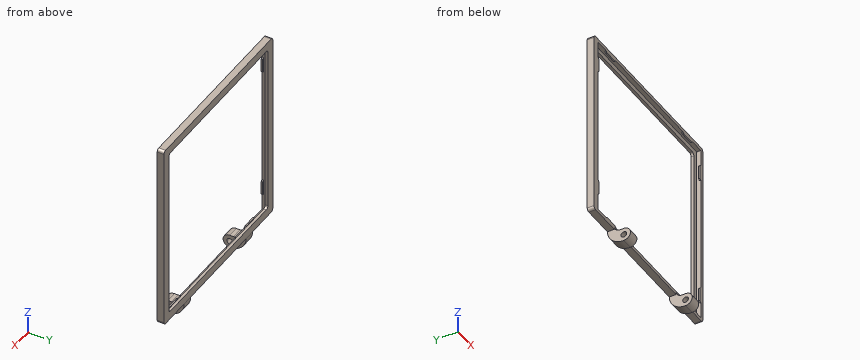
Autodesk Inventor part; units mm, degrees
ref_plane "YZ Plane" through (0, 0, 0) normal (1, 0, 0) x (0, 1, 0)
ref_plane "XZ Plane" through (0, 0, 0) normal (0, 1, 0) x (-1, 0, 0)
ref_plane "XY Plane" through (0, 0, 0) normal (0, 0, 1) x (1, 0, 0)
sketch "Boceto1" plane through (0, 0, 0) normal (0, 1, 0) x (-1, 0, 0)
  line L0 (2, 0) -> (132.4, 0)
  line L1 (134.4, -2) -> (134.4, -138)
  line L2 (132.4, -140) -> (2, -140)
  line L3 (0, -138) -> (0, -2)
  arc A0 (134.4, -2) -> (132.4, 0) centre (132.4, -2) ccw
  arc A1 (132.4, -140) -> (134.4, -138) centre (132.4, -138) ccw
  arc A2 (0, -138) -> (2, -140) centre (2, -138) ccw
  arc A3 (2, 0) -> (0, -2) centre (2, -2) ccw
  line L4 (126.4, -6) -> (8, -6)
  line L5 (6, -8) -> (6, -132)
  line L6 (8, -134) -> (126.4, -134)
  line L7 (128.4, -132) -> (128.4, -8)
  arc A4 (8, -6) -> (6, -8) centre (8, -8) ccw
  arc A5 (6, -132) -> (8, -134) centre (8, -132) ccw
  arc A6 (126.4, -134) -> (128.4, -132) centre (126.4, -132) ccw
  arc A7 (128.4, -8) -> (126.4, -6) centre (126.4, -8) ccw
  line L8 (67.2, -140) -> (67.2, 0) construction
  line L9 (134.4, -140) -> (109.4, -140) construction
  line L10 (109.4, -140) -> (101.4, -140) construction
  line L11 (101.4, -140) -> (101.4, -152)
  line L12 (101.4, -152) -> (109.4, -152)
  line L13 (109.4, -152) -> (109.4, -140)
  line L14 (0, -140) -> (25, -140) construction
  line L15 (25, -140) -> (33, -140) construction
  line L16 (33, -140) -> (33, -152)
  line L17 (33, -152) -> (25, -152)
  line L18 (25, -152) -> (25, -140)
  point P0 (0, 0)
  point P1 (134.4, 0)
  point P2 (25, -140)
  point P3 (101.4, -140)
  dimension "d0" = 134.4
  dimension "d1" = 140
  dimension "d2" = 2
  dimension "d3" = 6
  dimension "d4" = 2
  dimension "d7" = 25
  dimension "d8" = 8
  dimension "d9" = 12
extrude "Extrusión1" add sketch "Boceto1" along normal blind 5
sketch "Boceto2" plane through (0, 0, 0) normal (0, -1, 0) x (1, 0, 0)
  line L0 (-25, -140) -> (-25, -152)
  line L1 (-33, -140) -> (-101.4, -140)
  line L2 (-25, -152) -> (-33, -152)
  line L3 (-33, -152) -> (-33, -140)
  line L4 (-33, -140) -> (-25, -140)
  line L5 (-25, -140) -> (-25, -152)
  line L6 (-101.4, -152) -> (-109.4, -152)
  line L7 (-109.4, -152) -> (-101.4, -152)
  line L8 (-101.4, -152) -> (-101.4, -140)
  line L9 (-101.4, -140) -> (-109.4, -140)
  line L10 (-109.4, -140) -> (-109.4, -152)
  line L11 (-109.4, -140) -> (-101.4, -140)
  line L12 (-101.4, -140) -> (-101.4, -136)
  line L13 (-101.4, -136) -> (-109.4, -136)
  line L14 (-109.4, -136) -> (-109.4, -140)
  line L15 (-33, -140) -> (-25, -140)
  line L16 (-25, -140) -> (-25, -136)
  line L17 (-25, -136) -> (-33, -136)
  line L18 (-33, -136) -> (-33, -140)
  point P0 (0, 0)
  dimension "d18" = 4
  dimension "d19" = 8
  dimension "d20" = 4
extrude "Extrusión2" add sketch "Boceto2" along normal blind 18
sketch "Boceto3" plane through (-109.4, 5, -152) normal (-1, 0, 0) x (0, 0, 1)
  line L0 (14, -5) -> (12, -5) construction
  line L1 (0, -23) -> (0, 0)
  line L2 (12, -5) -> (0, -5) construction
  line L3 (0, -5) -> (0, -12) construction
  line L4 (12, -12) -> (12, -5) construction
  circle A0 centre (5, -12) radius 2.125
  circle A1 centre (5, -12) radius 4.875 construction
  arc A2 (0.125, -12) -> (9.875, -12) centre (5, -12) ccw
  line L5 (0.125, -12) -> (0.125, 0) construction
  line L6 (12, 0) -> (0, 0) construction
  line L7 (12, -5) -> (12, 0) construction
  line L8 (9.8743, -12.0803) -> (9.8743, -5) construction
  line L9 (12, -5) -> (5, -5) construction
  line L10 (5, -5) -> (5, -12) construction
  line L11 (5, -12) -> (12, -12) construction
  line L12 (12, -12) -> (12, -5) construction
  line L13 (14, -5) -> (14, -23) construction
  line L14 (16, -23) -> (0, -23)
  line L15 (12, -5) -> (14, -5) construction
  line L16 (14, -5) -> (14, -7) construction
  line L17 (14, -7) -> (12, -7) construction
  line L18 (12, -7) -> (12, -5) construction
  arc A3 (14, -5) -> (12, -7) centre (14, -7) ccw construction
  line L19 (14, 0) -> (150, 0)
  line L20 (12, 0) -> (14, 0)
  arc A4 (12, 0) -> (0.125, -12) centre (12, -11.8757) ccw
  line L21 (14, -5) -> (16, -5)
  arc A5 (14, -5) -> (9.8743, -9.1856) centre (14, -9.1261) ccw
  line L22 (9.8743, -12.0803) -> (9.8743, -9.1856)
  line L23 (0.125, 0) -> (14, 0)
  line L24 (14, 0) -> (14, -23)
  line L25 (14, -23) -> (0, -23)
  line L26 (16, -23) -> (14, -23)
  line L27 (14, -23) -> (14, -5)
  line L28 (14, -5) -> (16, -5)
  line L29 (16, -5) -> (16, -23)
  line L30 (0.125, 0) -> (-6.5711, 0)
  line L31 (-6.5711, 0) -> (-6.5711, -23)
  line L32 (-6.5711, -23) -> (16, -23)
  point P0 (152, -5)
  point P1 (9.8743, -9.1856)
  point P2 (9.8743, -12.0803)
  point P3 (0, -10.3846)
  point P4 (0, -13.125)
  point P5 (12, 0)
  point P6 (0, 0)
  point P7 (14, -5)
  point P8 (14, -5)
  dimension "d13" = 4.25
  dimension "d14" = 2.75
  dimension "d16" = 7
  dimension "d17" = 7
  dimension "d21" = 2
extrude "Extrusión3" cut sketch "Boceto3" against normal blind 150 contours L1 L30 L23 A4 A2 L22 A5 L24 L14 | L24 L21 L29 L14 | A0
sketch "Boceto4" plane through (0, 0, 0) normal (0, -1, 0) x (1, 0, 0)
  line L0 (0, 0) -> (-132, 0)
  line L1 (-132, 0) -> (-132, -140)
  line L2 (-132, -140) -> (0, -140)
  line L3 (0, -140) -> (0, 0)
  line L4 (-2.5, -2.5) -> (-129.5, -2.5)
  line L5 (-129.5, -2.5) -> (-129.5, -137.5)
  line L6 (-129.5, -137.5) -> (-2.5, -137.5)
  line L7 (-2.5, -137.5) -> (-2.5, -2.5)
  dimension "d27" = 132
  dimension "d28" = 140
  dimension "d29" = 2.5
extrude "Extrusión4" cut sketch "Boceto4" against normal blind 3 contours L7 L6 L5 L4
sketch "Boceto5" plane through (0, 0, 0) normal (0, -1, 0) x (1, 0, 0)
  line L0 (-129.5, -137.5) -> (-129.5, -2.5)
  line L1 (-2.5, -2.5) -> (-2.5, -137.5)
  line L2 (-129.5, -137.5) -> (-2.5, -137.5)
  line L3 (-2.5, -137.5) -> (-2.5, -2.5)
  line L4 (-2.5, -2.5) -> (-129.5, -2.5)
  line L5 (-129.5, -2.5) -> (-129.5, -137.5)
  line L6 (-2.5, -137.5) -> (-129.5, -137.5)
  line L7 (-66, -137.5) -> (-66, -2.5) construction
  line L8 (-33, -140) -> (-101.4, -140) construction
  line L9 (-2.5, -70) -> (-129.5, -70) construction
  line L10 (-118.5, -137.5) -> (-107.5, -137.5) construction
  line L11 (-118.5, -137.5) -> (-108.5, -137.5) construction
  line L12 (-108.5, -137.5) -> (-108.5, -136.5) construction
  line L13 (-108.5, -136.5) -> (-118.5, -136.5) construction
  line L14 (-118.5, -136.5) -> (-118.5, -137.5) construction
  line L15 (-118.5, -137.5) -> (-119.5, -137.5) construction
  line L16 (-119.5, -137.5) -> (-118.5, -136.5) construction
  line L17 (-108.5, -137.5) -> (-107.5, -137.5) construction
  line L18 (-107.5, -137.5) -> (-108.5, -136.5) construction
  line L19 (-107.5, -137.5) -> (-108.5, -136.5)
  line L20 (-118.5, -136.5) -> (-119.5, -137.5)
  line L21 (-118.5, -136.5) -> (-108.5, -136.5)
  line L22 (-129.5, -124.5) -> (-128.5, -124.5) construction
  line L23 (-128.5, -124.5) -> (-128.5, -114.5) construction
  line L24 (-128.5, -114.5) -> (-129.5, -114.5) construction
  line L25 (-129.5, -114.5) -> (-129.5, -124.5) construction
  line L26 (-129.5, -124.5) -> (-129.5, -125.5) construction
  line L27 (-129.5, -125.5) -> (-128.5, -124.5) construction
  line L28 (-129.5, -114.5) -> (-129.5, -113.5) construction
  line L29 (-129.5, -113.5) -> (-128.5, -114.5) construction
  line L30 (-129.5, -125.5) -> (-128.5, -124.5)
  line L31 (-128.5, -114.5) -> (-128.5, -124.5)
  line L32 (-129.5, -113.5) -> (-128.5, -114.5)
  line L33 (-107.5, -137.5) -> (-119.5, -137.5)
  line L34 (-129.5, -125.5) -> (-129.5, -113.5)
  line L35 (-118.5, -2.5) -> (-107.5, -2.5) construction
  line L36 (-118.5, -2.5) -> (-108.5, -2.5) construction
  line L37 (-108.5, -2.5) -> (-108.5, -3.5) construction
  line L38 (-108.5, -3.5) -> (-118.5, -3.5) construction
  line L39 (-118.5, -3.5) -> (-118.5, -2.5) construction
  line L40 (-118.5, -2.5) -> (-119.5, -2.5) construction
  line L41 (-119.5, -2.5) -> (-118.5, -3.5) construction
  line L42 (-108.5, -2.5) -> (-107.5, -2.5) construction
  line L43 (-107.5, -2.5) -> (-108.5, -3.5) construction
  line L44 (-107.5, -2.5) -> (-108.5, -3.5)
  line L45 (-118.5, -3.5) -> (-119.5, -2.5)
  line L46 (-118.5, -3.5) -> (-108.5, -3.5)
  line L47 (-129.5, -15.5) -> (-128.5, -15.5) construction
  line L48 (-128.5, -15.5) -> (-128.5, -25.5) construction
  line L49 (-128.5, -25.5) -> (-129.5, -25.5) construction
  line L50 (-129.5, -25.5) -> (-129.5, -15.5) construction
  line L51 (-129.5, -15.5) -> (-129.5, -14.5) construction
  line L52 (-129.5, -14.5) -> (-128.5, -15.5) construction
  line L53 (-129.5, -25.5) -> (-129.5, -26.5) construction
  line L54 (-129.5, -26.5) -> (-128.5, -25.5) construction
  line L55 (-129.5, -14.5) -> (-128.5, -15.5)
  line L56 (-128.5, -25.5) -> (-128.5, -15.5)
  line L57 (-129.5, -26.5) -> (-128.5, -25.5)
  line L58 (-107.5, -2.5) -> (-119.5, -2.5)
  line L59 (-129.5, -14.5) -> (-129.5, -26.5)
  line L60 (-2.5, -137.5) -> (-2.5, -2.5)
  line L61 (-2.5, -2.5) -> (-2.5, -137.5)
  line L62 (-13.5, -137.5) -> (-24.5, -137.5) construction
  line L63 (-13.5, -137.5) -> (-23.5, -137.5) construction
  line L64 (-23.5, -137.5) -> (-23.5, -136.5) construction
  line L65 (-23.5, -136.5) -> (-13.5, -136.5) construction
  line L66 (-13.5, -136.5) -> (-13.5, -137.5) construction
  line L67 (-13.5, -137.5) -> (-12.5, -137.5) construction
  line L68 (-12.5, -137.5) -> (-13.5, -136.5) construction
  line L69 (-23.5, -137.5) -> (-24.5, -137.5) construction
  line L70 (-24.5, -137.5) -> (-23.5, -136.5) construction
  line L71 (-24.5, -137.5) -> (-23.5, -136.5)
  line L72 (-13.5, -136.5) -> (-12.5, -137.5)
  line L73 (-13.5, -136.5) -> (-23.5, -136.5)
  line L74 (-2.5, -124.5) -> (-3.5, -124.5) construction
  line L75 (-3.5, -124.5) -> (-3.5, -114.5) construction
  line L76 (-3.5, -114.5) -> (-2.5, -114.5) construction
  line L77 (-2.5, -114.5) -> (-2.5, -124.5) construction
  line L78 (-2.5, -124.5) -> (-2.5, -125.5) construction
  line L79 (-2.5, -125.5) -> (-3.5, -124.5) construction
  line L80 (-2.5, -114.5) -> (-2.5, -113.5) construction
  line L81 (-2.5, -113.5) -> (-3.5, -114.5) construction
  line L82 (-2.5, -125.5) -> (-3.5, -124.5)
  line L83 (-3.5, -114.5) -> (-3.5, -124.5)
  line L84 (-2.5, -113.5) -> (-3.5, -114.5)
  line L85 (-24.5, -137.5) -> (-12.5, -137.5)
  line L86 (-2.5, -125.5) -> (-2.5, -113.5)
  line L87 (-3.5, -25.5) -> (-2.5, -25.5) construction
  line L88 (-2.5, -26.5) -> (-3.5, -25.5) construction
  line L89 (-2.5, -26.5) -> (-3.5, -25.5)
  line L90 (-2.5, -15.5) -> (-3.5, -15.5) construction
  line L91 (-2.5, -25.5) -> (-2.5, -15.5) construction
  line L92 (-2.5, -14.5) -> (-3.5, -15.5) construction
  line L93 (-2.5, -14.5) -> (-3.5, -15.5)
  line L94 (-2.5, -14.5) -> (-2.5, -26.5)
  line L95 (-2.5, -25.5) -> (-2.5, -26.5) construction
  line L96 (-3.5, -15.5) -> (-3.5, -25.5) construction
  line L97 (-3.5, -25.5) -> (-3.5, -15.5)
  line L98 (-2.5, -15.5) -> (-2.5, -14.5) construction
  line L99 (-13.5, -2.5) -> (-24.5, -2.5) construction
  line L100 (-13.5, -2.5) -> (-12.5, -2.5) construction
  line L101 (-12.5, -2.5) -> (-13.5, -3.5) construction
  line L102 (-13.5, -3.5) -> (-12.5, -2.5)
  line L103 (-23.5, -3.5) -> (-13.5, -3.5) construction
  line L104 (-13.5, -3.5) -> (-23.5, -3.5)
  line L105 (-13.5, -2.5) -> (-23.5, -2.5) construction
  line L106 (-23.5, -2.5) -> (-23.5, -3.5) construction
  line L107 (-24.5, -2.5) -> (-12.5, -2.5)
  line L108 (-23.5, -2.5) -> (-24.5, -2.5) construction
  line L109 (-24.5, -2.5) -> (-23.5, -3.5) construction
  line L110 (-24.5, -2.5) -> (-23.5, -3.5)
  line L111 (-13.5, -3.5) -> (-13.5, -2.5) construction
  point P0 (0, 0)
  point P1 (-101.4, 0)
  point P2 (-30.6, 0)
  dimension "d32" = 11
  dimension "d33" = 13
  dimension "d36" = 10
  dimension "d37" = 1
  dimension "d38" = 1
  dimension "d40" = 1
  dimension "d41" = 1
  dimension "d42" = 10
  dimension "d43" = 1
  dimension "d44" = 1
extrude "Extrusión5" add sketch "Boceto5" against normal blind 1 contours L0 L32 L31 L30 | L20 L21 L19 L2 | L0 L55 L56 L57 | L71 L73 L72 L2 | L4 L44 L46 L45 | L82 L83 L84 L1 | L4 L102 L104 L110 | L89 L97 L93 L1
Source: CAD feature listing. Evaluate the final solid. Frame: model axes, mm. Round coordinates to 2 decimals unless told otherwise and drop trailing zeros. Loops run counter-clockwise (first coordinate to the right, second up) from the corner with the lowest first, then second, coordinate; pieces in that order, holes last.
1. Section query C-C on x = -66. Output: boundary loops of the cut face in (y, z).
2. Section query A-A on z = -22.5. Output: boundary loops of the cut face in (x, y).
3. Ray query, L1, parallel to Z at x = -11, y = 4.25; L2, parallel to X at y = 1, z = -62.5; L3, parallel to X at y = 3.25, z = -32.5. Return the intervals inside material, ascending.
4. Section query D-D on z = -147. Output: boundary loops of the cut face in (x, y) (3 decimals), and give its area (3 significant figures).
5. Contact query for flat-ended pins moving along their axis: pin 1 (7 mm diameter, centred on y = -3.5, z = -142.5, fed in from -X); pin 2 (0.8 mm diameter, centred on x = -27, y = -5.5, fed in from +Z); pin 3 (1.5 mm diameter, centred on x = -70.5, y = 1.5, fed in from -Z). Output: stop coordinate, or through.
Answers below:
1. outline: (0, -140) - (5, -140) - (5, -134) - (3, -134) - (3, -137.5) - (0, -137.5) - close; (0, -2.5) - (3, -2.5) - (3, -6) - (5, -6) - (5, 0) - (0, 0) - close
2. outline: (-134.4, 0) - (-128.5, 0) - (-128.5, 1) - (-129.5, 1) - (-129.5, 3) - (-128.4, 3) - (-128.4, 5) - (-134.4, 5) - close; (-6, 3) - (-2.5, 3) - (-2.5, 1) - (-3.5, 1) - (-3.5, 0) - (0, 0) - (0, 5) - (-6, 5) - close
3. L1: z = -140 to -134, -6 to 0
3. L2: x = -134.4 to -129.5, -2.5 to 0
3. L3: x = -134.4 to -128.4, -6 to 0
4. outline: (-109.4, -11.875) - (-101.4, -11.875) - (-101.4, -9.125) - (-109.4, -9.125) - close; (-109.4, -4.875) - (-101.4, -4.875) - (-101.4, 2.718) - (-109.4, 2.718) - close; (-33, -11.875) - (-25, -11.875) - (-25, -9.125) - (-33, -9.125) - close; (-33, -4.875) - (-25, -4.875) - (-25, 2.718) - (-33, 2.718) - close
4. area: 165 mm2
5. pin 1: stops at x = -109.4
5. pin 2: stops at z = -142.13
5. pin 3: stops at z = -140
